The model under review builds one solid part; all positions refer to its coordinate system, in mm. A direction names the side the tool comes from. Round coordinates to 2 decimals unless told otherwise and drop trailing zeros. Order: outer loops, then holes, each group sorted by start corner. A loop starts at its lowest first (then second) coordinate and runs counter-clockwise, first axis right, second up. Notation, with made-up numbers: M 89,89.25 L 116,89.25 A26 cw 116,123.25 Z; hole C 24,81 d5. An arc over 180 degrees is marked long. Answer as a JSON object with one key per item and string values. Group by question number.
1. Add section D-D on y = -0.25. State the section outline as (x, z) points (3 decimals).
2. Add section C-C on z = 0. State the section outline as (x, y) points, and give its area (3 significant figures).
3. Machinability: for faces 1 (the face through (-2, 0, 0)), 2 (the face through (0, 1, -3)), which of the approach directions +Z, -Z, +X, -X, +Y, -Y give a long, thin tool a straight path to every point of the face, cutting with its end or side? Answer none if there is none.
4. Clearance check with flat-ended pins moving along their axes: P1, Ø0.6, axis at x = 2, z = -0.5, coming from the -Y side; P2, Ø1.3, axis at x = -2, z = -0.5, coming from the -Y side. State where each tip first meets the part, or that it passes through.
5. Add section B-B on y = 3. State the section outline as (x, z) points, and give its area (3 significant figures).
6. Add section A-A on x = 0. State the section outline as (y, z) points, and give its area (3 significant figures).
7. To check wall thickness, follow probe 1 along X at (y, z) = (2, 0); probe 2 along Z at (x, y) = (-0.8, 0.75); probe 3 along Z at (x, y) = (0, 4.75). State the ranges of each line that lie inside material, in increasing order. Write a range as [from, to].
8. Mouldability with a two-part tool opening along X and no side actions: class faces 3 (the face through (0, 8, 1.3)), 4 (the face through (2.715, 0.395, 2.699)), 5 (the face through (0.01, -3.45, 2.53)), 6 (the face through (-2.699, 0.395, 2.715)) as released by +X, released by -X, zero draft, split by the parting line, or undercut.
```python
from build123d import *

# Parameters (mm, degrees)
SKETCH2_W           = 6
SKETCH2_H           = 6
BOSS_EXTRUDE1_DEPTH = 8
SKETCH7_W           = 6
SKETCH7_H           = 6
BOSS_EXTRUDE2_DEPTH = 7
FILLET1_R           = 1


with BuildPart() as part:
    # Sketch2 → Boss-Extrude1 (new body)
    with BuildSketch(Plane(origin=(0, 0, 0), x_dir=(1, 0, 0), z_dir=(0, 1, 0))):
        Rectangle(SKETCH2_W, SKETCH2_H)
        with BuildLine():
            Line((-1.178982612, -1.14), (1.178982612, -1.14))
            ThreePointArc((1.178982612, -1.14), (0, 1.64), (-1.178982612, -1.14))
        make_face(mode=Mode.SUBTRACT)
    extrude(amount=BOSS_EXTRUDE1_DEPTH)

    # Sketch7 → Boss-Extrude2 (add)
    with BuildSketch(Plane(origin=(0, 0, 0), x_dir=(-1, 0, 0), z_dir=(0, -1, 0))):
        Rectangle(SKETCH7_W, SKETCH7_H)
        with BuildLine():
            Line((-2.35, -0.935), (-1.435, -0.935))
            ThreePointArc((-1.435, -0.935), (-1.081446609, -1.081446609), (-0.935, -1.435))
            Line((-0.935, -1.435), (-0.935, -2.35))
            ThreePointArc((-0.935, -2.35), (0, -2.529174767), (0.935, -2.35))
            Line((0.935, -2.35), (0.935, -1.435))
            ThreePointArc((0.935, -1.435), (1.081446609, -1.081446609), (1.435, -0.935))
            Line((1.435, -0.935), (2.35, -0.935))
            ThreePointArc((2.35, -0.935), (2.529174767, 0), (2.35, 0.935))
            Line((2.35, 0.935), (1.435, 0.935))
            ThreePointArc((1.435, 0.935), (1.081446609, 1.081446609), (0.935, 1.435))
            Line((0.935, 1.435), (0.935, 2.35))
            ThreePointArc((0.935, 2.35), (0, 2.529174767), (-0.935, 2.35))
            Line((-0.935, 2.35), (-0.935, 1.435))
            ThreePointArc((-0.935, 1.435), (-1.081446609, 1.081446609), (-1.435, 0.935))
            Line((-1.435, 0.935), (-2.35, 0.935))
            ThreePointArc((-2.35, 0.935), (-2.529174767, 0), (-2.35, -0.935))
        make_face(mode=Mode.SUBTRACT)
    extrude(amount=BOSS_EXTRUDE2_DEPTH)

    # Fillet1
    fillet1_edges = [part.edges().sort_by_distance(p)[0] for p in [
        (3, 0.5, 3),
        (-3, 0.5, 3),
        (-3, 0.5, -3),
        (3, 0.5, -3),
    ]]
    fillet(fillet1_edges, radius=FILLET1_R)


solid = part.part
```
Recorded:
{
 "1": {"outline": "M -3,-2 A1 ccw -2,-3 L 2,-3 A1 ccw 3,-2 L 3,2 A1 ccw 2,3 L -2,3 A1 ccw -3,2 Z; hole M -2.35,-0.935 L -1.435,-0.935 A0.5 cw -0.935,-1.435 L -0.935,-2.35 A2.529 ccw 0.935,-2.35 L 0.935,-1.435 A0.5 cw 1.435,-0.935 L 2.35,-0.935 A2.529 ccw 2.35,0.935 L 1.435,0.935 A0.5 cw 0.935,1.435 L 0.935,2.35 A2.529 ccw -0.935,2.35 L -0.935,1.435 A0.5 cw -1.435,0.935 L -2.35,0.935 A2.529 ccw Z"},
 "2": {"outline": "M -3,-7 L -2.53,-7 L -2.53,0 L -1.64,0 L -1.64,8 L -3,8 Z; M 1.64,0 L 2.53,0 L 2.53,-7 L 3,-7 L 3,8 L 1.64,8 Z", "area": "28.4 mm²"},
 "3": {"face 1": "-Y", "face 2": "-Z, +X, -X, +Y, -Y"},
 "4": {"P1": "stops at y = 0", "P2": "stops at y = -7"},
 "5": {"outline": "M -3,-2 A1 ccw -2,-3 L 2,-3 A1 ccw 3,-2 L 3,2 A1 ccw 2,3 L -2,3 A1 ccw -3,2 Z; hole M -1.18,1.14 A1.64 ccw long 1.18,1.14 Z", "area": "27.5 mm²"},
 "6": {"outline": "M -7,-3 L 8,-3 L 8,-1.64 L 0,-1.64 L 0,-2.53 L -7,-2.53 Z; M -7,2.53 L 0,2.53 L 0,1.14 L 8,1.14 L 8,3 L -7,3 Z", "area": "32.4 mm²"},
 "7": {"probe 1": "x = [-3, -1.64], [1.64, 3]", "probe 2": "z = [-3, -1.43], [1.14, 3]", "probe 3": "z = [-3, -1.64], [1.14, 3]"},
 "8": {"face 3": "zero draft", "face 4": "released by +X", "face 5": "undercut", "face 6": "released by -X"}
}
